The figure shows three views and two pictorial views of one solid part (mm, origin at its lowest corner). Answer the questions. A direction names the side the tool comes from. Give positions to 0.01 mm unless a question says otherwise; leave off trailing zeros. Loops run counter-clockwise (first coordinate to the right, second up) from the corner with the lowest first, then second, coordinate; pieces in that order, holes last. Notation, with made-up numbers: (79.5, 59) - (120.5, 59) arc R35 cw to (120.5, 93) - close; hole circle Ø1 at (78, 70.5). An arc over 180 degrees is marked (long way). Write item = value, one per line.
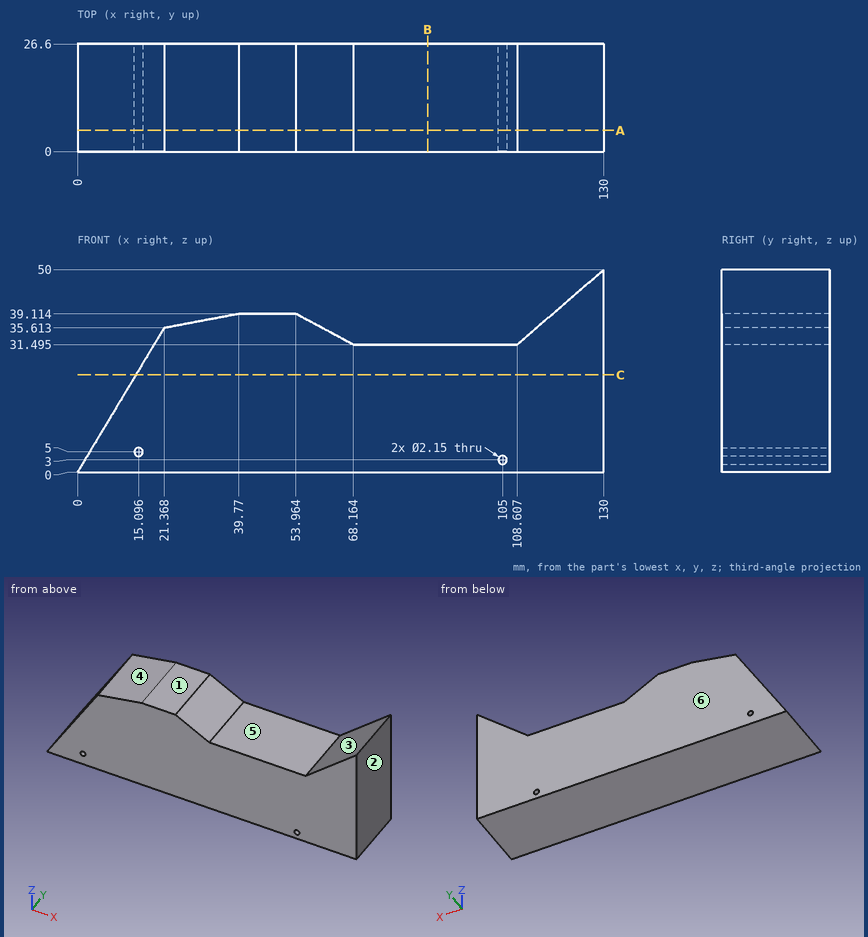
1) A cutting plane is placed at B-B on x = 86.5. Determine the outline of the cut face in (y, z) (1 decimal).
Output:
outline = (0, 0) - (26.6, 0) - (26.6, 31.5) - (0, 31.5) - close
2) A tool of negligible diameter and unlimited length cuts with its end or side. For the marked faces 5 and 6, from which of +Z, -Z, +X, -X, +Y, -Y can it reach the whole face along a straight path? Write none if from no direction.
Output:
face_5 = +Z, +Y, -Y
face_6 = +Z, -Z, +X, -X, +Y
3) Each of these flat-tipped pins is pushed along its axis until it touches: P1, Ø5, axis at y = 3.5, z = 10, coming from the -X side; P2, Ø8, axis at x = 71, y = 16, coming from the +Z side; P3, Ø10, axis at y = 3, z = 19, coming from the -X side; P4, Ø1.3, axis at x = 105, z = 3, coming from the -Y side. Where does it stop, or does it pass through?
Output:
P1 = 4.5
P2 = 32.12
P3 = 8.4
P4 = through
4) A cutting plane is placed at A-A on y = 5.25. Give the number of separate pieces and of enclosed holes in the cut face, then the cut area to 3 significant figures.
Output:
separate_pieces = 1
enclosed_holes = 2
area = 4,260 mm²
5) Find the intervals of material crossed by probe 1 along Z at (x, y) = (105, 15) (1 decimal); probe 2 along Z at (x, y) = (43.5, 5) (1 decimal); probe 3 along Z at (x, y) = (82, 12.25) (1 decimal), in increasing order.
Output:
probe_1 = 0 to 1.9, 4.1 to 31.5
probe_2 = 0 to 39.1
probe_3 = 0 to 31.5
6) A cutting plane is placed at C-C on z = 24. Determine the outline of the cut face in (x, y).
Output:
outline = (14.4, 0) - (130, 0) - (130, 26.6) - (14.4, 26.6) - close
7) The mould has two halves that part along X. Classify the marked faces 1, 2, 3 and 4: pulls with the +X half, pulls with the -X half, needs draft (parallel to the pull), parting line crosses it, or undercut.
Output:
face_1 = needs draft
face_2 = pulls with the +X half
face_3 = undercut
face_4 = pulls with the -X half
